```python
from build123d import *

# Parameters (mm, degrees)
SKETCH_1_W          = 74
SKETCH_1_H          = 14.8
EXTRUDE_1_DEPTH     = 14.8
SKETCH_2_W          = 10.4
SKETCH_2_H          = 10.4
CUT_EXTRUDE_1_DEPTH = 30
SKETCH_3_R          = 3.9
EXTRUDE_2_DEPTH     = 15
SKETCH_4_R          = 3.9
EXTRUDE_3_DEPTH     = 13
CHAMFER_1_SIZE      = 5
SKETCH_8_R          = 1.45
CUT_EXTRUDE_4_DEPTH = 43.8
SKETCH_9_W          = 7.8
SKETCH_9_H          = 7.8
SKETCH_9_R          = 1.5
EXTRUDE_4_DEPTH     = 3.55
SKETCH_10_W         = 7.8
SKETCH_10_H         = 7.8
EXTRUDE_5_DEPTH     = 3.55
SKETCH1_R           = 1.6
CUT_EXTRUDE1_DEPTH  = 30.8
SKETCH2_R           = 1.5
CUT_EXTRUDE2_DEPTH  = 43.8


with BuildPart() as part:
    # Эскиз1 → Бобышка-Вытянуть1 (new body)
    with BuildSketch(Plane(origin=(0, 0, 0), x_dir=(0, 0, -1), z_dir=(1, 0, 0))):
        Rectangle(SKETCH_1_W, SKETCH_1_H)
    extrude(amount=EXTRUDE_1_DEPTH)

    # Эскиз2 → Вырез-Вытянуть1 (cut)
    with BuildSketch(Plane(origin=(0, 0, -37), x_dir=(-1, 0, 0), z_dir=(0, 0, -1))):
        with Locations((-7.4, 0)):
            Rectangle(SKETCH_2_W, SKETCH_2_H)
    extrude(amount=-CUT_EXTRUDE_1_DEPTH, mode=Mode.SUBTRACT)

    # Эскиз3 → Бобышка-Вытянуть2 (add)
    with BuildSketch(Plane(origin=(14.8, 0, 0), x_dir=(0, 0, -1), z_dir=(1, 0, 0))):
        with Locations(Location((-33.1, 0, 0), (0, 0, 180))):  # turned: the seam where the file's is
            Circle(SKETCH_3_R)
    extrude(amount=EXTRUDE_2_DEPTH)

    # Эскиз4 → Бобышка-Вытянуть3 (add)
    with BuildSketch(Plane.ZY):
        with Locations((33.1, 0)):
            Circle(SKETCH_4_R)
    extrude(amount=EXTRUDE_3_DEPTH)

    # Фаска1
    chamfer_1_edges = [part.edges().sort_by_distance(p)[0] for p in [
        (7.4, 7.4, 37),
        (7.4, -7.4, 37),
    ]]
    chamfer(chamfer_1_edges, length=CHAMFER_1_SIZE)

    # Эскиз8 → Вырез-Вытянуть4 (cut, through all)
    with BuildSketch(Plane(origin=(29.8, 0, 0), x_dir=(0, 0, -1), z_dir=(1, 0, 0))):
        with Locations((-33.1, 0)):
            Circle(SKETCH_8_R)
    extrude(amount=-CUT_EXTRUDE_4_DEPTH, mode=Mode.SUBTRACT)

    # Эскиз9 → Бобышка-Вытянуть4 (add)
    with BuildSketch(Plane.ZY):
        with Locations((33.1, 0)):
            Rectangle(SKETCH_9_W, SKETCH_9_H)
        with Locations((33.1, 0)):
            Circle(SKETCH_9_R, mode=Mode.SUBTRACT)
    extrude(amount=EXTRUDE_4_DEPTH)

    # Эскиз10 → Бобышка-Вытянуть5 (add)
    with BuildSketch(Plane(origin=(14.8, 0, 0), x_dir=(0, 0, -1), z_dir=(1, 0, 0))):
        with Locations((-33.1, 0)):
            Rectangle(SKETCH_10_W, SKETCH_10_H)
    extrude(amount=EXTRUDE_5_DEPTH)

    # Sketch1 → Cut-Extrude1 (cut, through all)
    with BuildSketch(Plane.ZY):
        with Locations((-32, 0)):
            Circle(SKETCH1_R)
        with Locations((-22, 0)):
            Circle(SKETCH1_R)
    extrude(amount=-CUT_EXTRUDE1_DEPTH, mode=Mode.SUBTRACT)

    # Sketch2 → Cut-Extrude2 (cut, through all)
    with BuildSketch(Plane(origin=(29.8, 0, 0), x_dir=(0, 0, -1), z_dir=(1, 0, 0))):
        with Locations((-33.1, 0)):
            Circle(SKETCH2_R)
    extrude(amount=-CUT_EXTRUDE2_DEPTH, mode=Mode.SUBTRACT)


solid = part.part
```
The model under review builds one solid part; all positions refer to its coordinate system, in mm. A direction names the side the tool comes from. Give positions to 0.01 mm unless a question says otherwise; leave off trailing zeros. Write each loop counter-clockwise with the first axis right and the second up, starting at its lowest first coordinate (ties: lowest second). Pieces come first, ordered by that corner, then holes.
(1) Consider section D-D, the plane z = 4.5. Give the boundary of the cut face in (x, y), and give its area (3 significant figures).
(2) For P1, Ø1.8, axis at x = 16.5, z = 32, coming from the -Y side; P2, Ø0.5, axis at y = 3.5, z = 36, coming from the -X side; P3, Ø1.5, axis at y = 0.5, z = 25.5, coming from the +X side, all flat-tipped, find the tip position at first contact; note any pin that passes through.
(3) Consider section B-B, the plane x = 14. Give the boundary of the cut face in (y, z), and give its area (3 significant figures).
(4) To check wall thickness, follow L1, parallel to Y at x = 13.2, z = -22; L2, parallel to Y at x = 18, z = 33.1; L3, parallel to X at y = 2.25, z = -33.5. State the ranges of each line that lie inside material, in increasing order.
(5) The part is to be moulded in two halves that separate along Y. For faces 5 (the flat face through (-2, 3.9, 33)), 6 (the cylindrical face through (13.685, 0.481, -20.474)), 7 (the flat face through (-2, 0, 29.2)), say which applies: released by +Y, released by -Y, zero draft, split by the parting line, or undercut.
(6) Consider section C-C, the plane x = 21.5. Give the boundary of the cut face in (y, z).
(7) Tool access review of faces 1 (the flat face through (-3.55, 3, 36)), 2 (the flat face through (-3.55, -3, 30)), 3 (the flat face through (7.3, 4.9, 34.5)), 4 (the flat face through (18.35, 3, 36)): name each direction out of +Z, -Z, +X, -X, +Y, -Y from which nothing blocks a thin tool from reaching the whole face with its end or side.
(8) Consider section A-A, the plane z = -22. Give the boundary of the cut face in (x, y).
Returned:
1. outline: (0, -7.4) - (14.8, -7.4) - (14.8, 7.4) - (0, 7.4) - close
1. area: 219 mm2
2. P1: stops at y = -3.9
2. P2: stops at x = -3.55
2. P3: stops at x = 14.8
3. outline: (-7.4, -37) - (7.4, -37) - (7.4, 32) - (2.4, 37) - (-2.4, 37) - (-7.4, 32) - close; hole circle Ø3.2 at (0, -32); hole circle Ø3.2 at (0, -22); hole circle Ø3 at (0, 33.1)
3. area: 1,050 mm2
4. L1: y = -7.4 to -1.6, 1.6 to 7.4
4. L2: y = -3.9 to -1.5, 1.5 to 3.9
4. L3: x = 0 to 2.2, 12.6 to 14.8
5. face 5: released by +Y
5. face 6: undercut
5. face 7: zero draft
6. outline: circle Ø7.8 at (0, 33.1); hole circle Ø3 at (0, 33.1)
7. face 1: +Z, -X, +Y
7. face 2: -Z, -X, -Y
7. face 3: +Z, +Y
7. face 4: +Z, +X, +Y
8. outline: (0, -7.4) - (14.8, -7.4) - (14.8, -1.6) - (12.6, -1.6) - (12.6, -5.2) - (2.2, -5.2) - (2.2, -1.6) - (0, -1.6) - close; (0, 1.6) - (2.2, 1.6) - (2.2, 5.2) - (12.6, 5.2) - (12.6, 1.6) - (14.8, 1.6) - (14.8, 7.4) - (0, 7.4) - close
